The listing builds one solid part. Answer for the finished solid, in the listing's coordinates (mm). Face numbers are marked on the shaded views. Coordinates: 2 decimals unless noted, no trailing zeros. Loops run counter-clockwise (first coordinate to the right, second up) from the corner with the lowest first, then second, coordinate; pieces in that order, holes last. Notation, with made-up numbers: (55, 24) -> (80, 24) arc R20 cw to (80, 42) -> close; hole circle Ø6 at (-10.75, 17.5). An arc over 180 degrees is marked (long way). Answer in a Markdown table with one row per item.
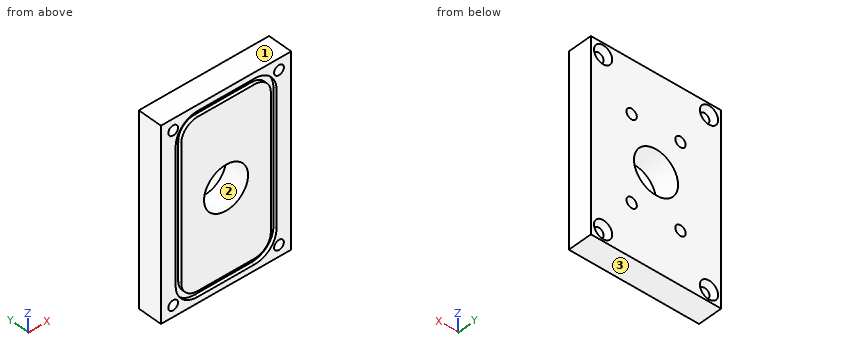
```python
from build123d import *

# Parameters (mm, degrees)
SKETCH1_W                                      = 50.8
SKETCH1_H                                      = 73.81875
BOSS_EXTRUDE1_DEPTH                            = 9.525
CSK_FOR_6_FLAT_HEAD_MACHINE_SCREW1_D           = 3.7973
CSK_FOR_6_FLAT_HEAD_MACHINE_SCREW1_CSINK_D     = 7.0866
CSK_FOR_6_FLAT_HEAD_MACHINE_SCREW1_CSINK_ANGLE = 82
CUT_EXTRUDE1_DASH_036_DEPTH                    = 1.3208
SKETCH5_R                                      = 8.5852
CUT_EXTRUDE1_DEPTH                             = 10.525
CIRPATTERN1_COUNT                              = 6


with BuildPart() as part:
    # Sketch1 → Boss-Extrude1 (new body)
    with BuildSketch(Plane(origin=(0, 0, 0), x_dir=(1, 0, 0), z_dir=(0, 1, 0))):
        Rectangle(SKETCH1_W, SKETCH1_H)
    extrude(amount=BOSS_EXTRUDE1_DEPTH)

    # CSK for #6 Flat Head Machine Screw1 (through all)
    with Locations(Plane(origin=(0, 9.525, 0), x_dir=(-1, 0, 0), z_dir=(0, 1, 0))):
        with Locations((20.6375, -32.54375), (-20.6375, -32.54375), (-20.6375, 32.54375), (20.6375, 32.54375)):
            CounterSinkHole(CSK_FOR_6_FLAT_HEAD_MACHINE_SCREW1_D / 2, CSK_FOR_6_FLAT_HEAD_MACHINE_SCREW1_CSINK_D / 2, counter_sink_angle=CSK_FOR_6_FLAT_HEAD_MACHINE_SCREW1_CSINK_ANGLE)

    # Sketch4 → Cut-Extrude1 - dash 036 (cut)
    with BuildSketch(Plane(origin=(0, 0, 0), x_dir=(-1, 0, 0), z_dir=(0, -1, 0))):
        with BuildLine():
            Line((-11.1125, 34.6075), (11.1125, 34.6075))
            ThreePointArc((11.1125, 34.6075), (17.147232113, 32.107832113), (19.6469, 26.0731))
            Line((19.6469, 26.0731), (19.6469, -26.0731))
            ThreePointArc((19.6469, -26.0731), (17.147232113, -32.107832113), (11.1125, -34.6075))
            Line((11.1125, -34.6075), (-11.1125, -34.6075))
            ThreePointArc((-11.1125, -34.6075), (-17.147232113, -32.107832113), (-19.6469, -26.0731))
            Line((-19.6469, -26.0731), (-19.6469, 26.0731))
            ThreePointArc((-19.6469, 26.0731), (-17.147232113, 32.107832113), (-11.1125, 34.6075))
        make_face()
        with BuildLine():
            Line((-11.1125, -32.4231), (11.1125, -32.4231))
            ThreePointArc((11.1125, -32.4231), (15.602628061, -30.563228061), (17.4625, -26.0731))
            Line((17.4625, -26.0731), (17.4625, 26.0731))
            ThreePointArc((17.4625, 26.0731), (15.602628061, 30.563228061), (11.1125, 32.4231))
            Line((11.1125, 32.4231), (-11.1125, 32.4231))
            ThreePointArc((-11.1125, 32.4231), (-15.602628061, 30.563228061), (-17.4625, 26.0731))
            Line((-17.4625, 26.0731), (-17.4625, -26.0731))
            ThreePointArc((-17.4625, -26.0731), (-15.602628061, -30.563228061), (-11.1125, -32.4231))
        make_face(mode=Mode.SUBTRACT)
    extrude(amount=-CUT_EXTRUDE1_DASH_036_DEPTH, mode=Mode.SUBTRACT)

    # Sketch5 → Cut-Extrude1 (cut, through all)
    with BuildSketch(Plane(origin=(0, 9.525, 0), x_dir=(1, 0, 0), z_dir=(0, 1, 0))):
        Circle(SKETCH5_R)
    extrude(amount=-CUT_EXTRUDE1_DEPTH, mode=Mode.SUBTRACT)

    # Sketch9 → #10-32 Tapped Hole2 (revolve, cut)
    with BuildSketch(Plane(origin=(9.525, 9.525, -16.497783942), x_dir=(0, 0, 1), z_dir=(1, 0, 0))):
        Polygon((0, 0), (0, 7.563317848), (2.0193, 6.35), (2.0193, 0), align=None)
    f_10_32_tapped_hole2 = revolve(axis=Axis((9.525, 15.875, -16.497783942), (0, -1, 0)), mode=Mode.SUBTRACT)

    # CirPattern1: #10-32 Tapped Hole2 ×6 about axis, 2 skipped
    cirpattern1_axis = Axis((0, 0, 0), (0, 1, 0))
    add([f_10_32_tapped_hole2.rotate(cirpattern1_axis, i * 360 / CIRPATTERN1_COUNT) for i in range(1, CIRPATTERN1_COUNT) if i not in (2, 5)], mode=Mode.SUBTRACT)


solid = part.part
```
Item 1: A cutting plane is placed at C-C, the plane y = 6.25. Count the separate pieces of the cut face and the enclosed holes in it, plus the area to 3 significant figures.
Findings below:
| item | result |
|---|---|
| separate pieces | 1 |
| enclosed holes | 9 |
| area | 3,420 mm2 |
Item 2: A cutting plane is placed at B-B, the plane x = 0. Determine the outline of the cut face in (y, z) (1 decimal), plus the area to 3 significant figures.
Findings below:
| item | result |
|---|---|
| outline | (0, -36.9) -> (9.5, -36.9) -> (9.5, -8.6) -> (0, -8.6) -> (0, -32.4) -> (1.3, -32.4) -> (1.3, -34.6) -> (0, -34.6) -> close; (0, 8.6) -> (9.5, 8.6) -> (9.5, 36.9) -> (0, 36.9) -> (0, 34.6) -> (1.3, 34.6) -> (1.3, 32.4) -> (0, 32.4) -> close |
| area | 534 mm2 |
Item 3: Find the intervals of material crossed by probe 1 along Z at (x, y) = (-10, 1); probe 2 along X at (y, z) = (0.75, 15); probe 3 along X at (y, z) = (6.5, -32), in increasing order.
Findings below:
| item | result |
|---|---|
| probe 1 | z = -36.91 to -34.61, -32.42 to 32.42, 34.61 to 36.91 |
| probe 2 | x = -25.4 to -19.65, -17.46 to 17.46, 19.65 to 25.4 |
| probe 3 | x = -25.4 to -22.46, -18.82 to 18.82, 22.46 to 25.4 |
Item 4: Flat-ended cylindrical pins translate along their axes: pin 1 Ø4.5 at (x, z) = (-20.64, 32.54) entering from +Y; pin 2 Ø6 at (x, z) = (20.64, 32.54) entering from +Y. Find the tip coordinate at first contact, or state that the pin passes through.
Findings below:
| item | result |
|---|---|
| pin 1 | stops at y = 8.04 |
| pin 2 | stops at y = 8.91 |
Item 5: A cutting plane is placed at A-A, the plane z = 0. Determine the outline of the cut face in (x, y) (1 decimal).
Findings below:
| item | result |
|---|---|
| outline | (-25.4, 0) -> (-19.6, 0) -> (-19.6, 1.3) -> (-17.5, 1.3) -> (-17.5, 0) -> (-8.6, 0) -> (-8.6, 9.5) -> (-25.4, 9.5) -> close; (8.6, 0) -> (17.5, 0) -> (17.5, 1.3) -> (19.6, 1.3) -> (19.6, 0) -> (25.4, 0) -> (25.4, 9.5) -> (8.6, 9.5) -> close |
Item 6: Determine the mould class of the marked faces 1, 2 and 3 for opening direction Z: +Z half, -Z half, draft (parallel to the pull), parting line (faces both ways), or undercut.
Findings below:
| item | result |
|---|---|
| face 1 | +Z half |
| face 2 | undercut |
| face 3 | -Z half |
